Autodesk Inventor part; units mm, degrees
sketch "Skizze1" plane through (0, 0, 0) normal (0, 0, 1) x (1, 0, 0)
  line L0 (-70, 70) -> (70, 70)
  line L1 (70, 70) -> (70, -70)
  line L2 (70, -70) -> (-70, -70)
  line L3 (-70, -70) -> (-70, 70)
  line L4 (0, 98) -> (0, -98)
  line L5 (-98, 0) -> (98, 0)
  point P0 (0, 0)
  dimension "d0" = 70
  dimension "d1" = 140
  dimension "d2" = 140
  dimension "d3" = 70
extrude "Extrusion1" add sketch "Skizze1" along normal blind 5
sketch "Skizze2" plane through (0, 0, 5) normal (0, 0, 1) x (1, 0, 0)
  point P0 (0, 0)
  point P1 (0, 0)
hole "Bohrung1" at (0, 0, 5) direction (0, 0, -1) diameter 6.7 depth 9.5
sketch "Skizze3" plane through (0, 0, 5) normal (0, 0, 1) x (1, 0, 0)
  circle A0 centre (0, 0) radius 3.35
  circle A1 centre (0, 0) radius 3.35
  line L0 (-70, 70) -> (-70, -70)
  line L1 (-70, -70) -> (70, -70)
  line L2 (70, -70) -> (70, 70)
  line L3 (70, 70) -> (-70, 70)
  circle A2 centre (0, 14) radius 2.35
  dimension "d13" = 14
  dimension "d14" = 4.7
extrude "Extrusion2" add sketch "Skizze3" along normal blind 4.3 contours A2
sketch "Skizze4" plane through (0, 0, 5) normal (0, 0, 1) x (1, 0, 0)
  circle A0 centre (0, 14) radius 2.35
  circle A1 centre (0, 0) radius 3.35
  line L0 (-70, 70) -> (-70, -70)
  line L1 (-70, -70) -> (70, -70)
  line L2 (70, -70) -> (70, 70)
  line L3 (70, 70) -> (-70, 70)
  line L4 (-98, 0) -> (98, 0)
  line L5 (0, 98) -> (0, -98)
  point P0 (-62, 62)
  point P1 (62, 62)
  point P2 (-62, -62)
  point P3 (62, -62)
  dimension "d17" = 62
  dimension "d18" = 62
  dimension "d21" = 124
  dimension "d24" = 124
hole "Bohrung2" at (-62, 62, 5) at (62, 62, 5) at (-62, -62, 5) at (62, -62, 5) direction (0, 0, -1) diameter 6.3 end through all
sketch "Skizze5" plane through (0, 0, 5) normal (0, 0, 1) x (1, 0, 0)
  circle A0 centre (-62, -62) radius 3.15
  circle A1 centre (-62, 62) radius 3.15
  circle A2 centre (62, 62) radius 3.15
  circle A3 centre (62, -62) radius 3.15
  circle A4 centre (0, 14) radius 2.35
  circle A5 centre (0, 0) radius 3.35
  line L0 (-70, 70) -> (-70, -70)
  line L1 (-70, -70) -> (70, -70)
  line L2 (70, -70) -> (70, 70)
  line L3 (70, 70) -> (-70, 70)
  line L4 (0, 98) -> (0, -98)
  line L5 (-98, 0) -> (98, 0)
  point P0 (-62, 0)
  point P1 (-62, 15.5)
  point P2 (-62, 31)
  point P3 (-62, 46.5)
  point P4 (0, 62)
  point P5 (-15.5, 62)
  point P6 (-31, 62)
  point P7 (-46.5, 62)
  dimension "d35" = 62
  dimension "d36" = 0
  dimension "d37" = 15.5
  dimension "d38" = 15.5
  dimension "d39" = 15.5
  dimension "d40" = 15.5
  dimension "d41" = 31
  dimension "d42" = 46.5
hole "Bohrung3" at (-62, 0, 5) at (-62, 15.5, 5) at (-62, 31, 5) at (-62, 46.5, 5) at (0, 62, 5) at (-15.5, 62, 5) at (-31, 62, 5) at (-46.5, 62, 5) direction (0, 0, -1) diameter 6.3 end through all
mirror "Spiegeln1" about plane through (0, 0, 0) normal (1, 0, 0) of "Bohrung3"
mirror "Spiegeln2" about plane through (0, 0, 0) normal (0, 1, 0) of "Bohrung3", "Spiegeln1"
equation "\"d0\" = 0.5 * d1"
equation "\"d3\" = 0.5 * d2"
properties part number "MessHalterV2"
For this review, take the finished solid that the model builds, in its own axes (mm). Coordinates: 2 decimals unless noted, no trailing zeros. Order: outer loops, then holes, each group sorted by start corner. A loop starts at its lowest first (then second) coordinate and runs counter-clockwise, first axis right, second up. Notation, with made-up numbers: (-13.5, -2) - (28.5, -2) arc R7 ccw to (28.5, 6) - close; hole circle Ø3 at (1.25, -4.75). An arc over 180 degrees is marked (long way). Answer as a JSON object with one key per item and string values. Group by question number.
1. The part is to be moulded in two halves that separate along Y. For faces 1 (the cylindrical face through (63.917, 64.5, 2.465)), 2 (the flat face through (-1, 70, 2)), 3 (the flat face through (-17, 1, 0)), say which applies: pulls with the +Y half, pulls with the -Y half, needs draft (parallel to the pull), parting line crosses it, or undercut.
2. For probe 1 along Y at (x, z) = (-15.5, 1.7); probe 2 along Y at (x, z) = (0, 1.25); probe 3 along X at (y, z) = (-32.5, 4.5), list the stretches that pass through material, from the lowest coordinate up.
3. We need section B-B on x = 46.5. State the section outline as (y, z) points.
4. Clearance check with flat-ended pins moving along their axes: P1, Ø8, axis at x = -15.5, y = 62, coming from the +Z side; P2, Ø5.5, axis at x = -62, y = 46.5, coming from the +Z side. State where each tip first meets the part, or that it passes through.
5. We need section A-A on y = 0. State the section outline as (x, z) points.
6. We need section D-D on z = 7.25. State the section outline as (x, y) points, then the cut area to 3 significant figures.
Final values:
{
 "1": {"face 1": "undercut", "face 2": "pulls with the +Y half", "face 3": "needs draft"},
 "2": {"probe 1": "-70 to -65.15, -58.85 to 58.85, 65.15 to 70", "probe 2": "-70 to -65.15, -58.85 to -3.35, 3.35 to 58.85, 65.15 to 70", "probe 3": "-70 to -64.77, -59.23 to 59.23, 64.77 to 70"},
 "3": {"outline": "(-70, 0) - (-65.15, 0) - (-65.15, 5) - (-70, 5) - close; (-58.85, 0) - (58.85, 0) - (58.85, 5) - (-58.85, 5) - close; (65.15, 0) - (70, 0) - (70, 5) - (65.15, 5) - close"},
 "4": {"P1": "z = 5", "P2": "through"},
 "5": {"outline": "(-70, 0) - (-65.15, 0) - (-65.15, 5) - (-70, 5) - close; (-58.85, 0) - (-3.35, 0) - (-3.35, 5) - (-58.85, 5) - close; (3.35, 0) - (58.85, 0) - (58.85, 5) - (3.35, 5) - close; (65.15, 0) - (70, 0) - (70, 5) - (65.15, 5) - close"},
 "6": {"outline": "circle Ø4.7 at (0, 14)", "area": "17.3 mm²"}
}
